Geometry check sheet. Reference: the model listing, model coordinates, mm. A direction names the side the tool comes from. Round coordinates to 2 decimals unless told otherwise and drop trailing zeros. Loops run counter-clockwise (first coordinate to the right, second up) from the corner with the lowest first, then second, coordinate; pieces in that order, holes last.
Autodesk Inventor part; units mm, degrees
ref_plane "YZ Plane" through (0, 0, 0) normal (1, 0, 0) x (0, 1, 0)
ref_plane "XZ Plane" through (0, 0, 0) normal (0, 1, 0) x (-1, 0, 0)
ref_plane "XY Plane" through (0, 0, 0) normal (0, 0, 1) x (1, 0, 0)
sketch "スケッチ1" plane through (0, 0, 0) normal (0, 0, 1) x (1, 0, 0)
  line L0 (0, 0) -> (80, 0)
  line L1 (80, 0) -> (80, 40)
  line L2 (80, 40) -> (0, 40)
  line L3 (0, 40) -> (0, 0)
  dimension "d0" = 80
  dimension "d1" = 40
extrude "押し出し1" add sketch "スケッチ1" along normal blind 40
sketch "スケッチ2" plane through (80, 0, 0) normal (1, 0, 0) x (0, 0, -1)
  line L0 (0, 40) -> (-40, 40)
  line L1 (-37, 40) -> (-3, 40)
  line L2 (-3, 40) -> (-3, 3)
  line L3 (-3, 3) -> (-37, 3)
  line L4 (-37, 3) -> (-37, 40)
  line L5 (-40, 0) -> (-40, 40)
  line L6 (0, 0) -> (0, 40)
  line L7 (0, 0) -> (-40, 0)
  dimension "d4" = 3
  dimension "d5" = 3
  dimension "d6" = 3
extrude "押し出し2" cut sketch "スケッチ2" against normal through all contours L2 L3 L4 L0
sketch "スケッチ3" plane through (0, 0, 40) normal (0, 0, 1) x (1, 0, 0)
  line L0 (0, 40) -> (80, 40)
  line L1 (40, 40) -> (40, 0)
  point P0 (0, 0)
  point P1 (20, 35)
  point P2 (60, 35)
  dimension "d9" = 5
  dimension "d10" = 20
hole "穴1" at (20, 35, 40) at (60, 35, 40) direction (0, 0, -1) diameter 6 end through all
sketch "スケッチ4" plane through (0, 0, 40) normal (0, 0, 1) x (1, 0, 0)
  line L0 (0, 40) -> (80, 40)
  line L1 (40, 40) -> (40, 0)
  point P0 (0, 0)
  point P1 (34, 30)
  point P2 (46, 30)
  dimension "d18" = 6
  dimension "d19" = 10
hole "穴2" at (34, 30, 40) at (46, 30, 40) direction (0, 0, -1) diameter 2.4 end through all
sketch "スケッチ5" plane through (0, 0, 0) normal (0, -1, 0) x (1, 0, 0)
  line L0 (80, 40) -> (0, 40)
  line L1 (40, 40) -> (40, 10)
  point P0 (0, 0)
sketch "スケッチ6" plane through (0, 0, 40) normal (0, 0, 1) x (1, 0, 0)
  line L0 (80, 40) -> (0, 40)
  line L1 (40, 40) -> (40, 0)
  line L2 (0, 0) -> (80, 0)
  circle A0 centre (20, 35) radius 3
  point P0 (20, 5)
  point P1 (60, 5)
  dimension "d27" = 20
  dimension "d28" = 30
hole "穴3" at (20, 5, 40) at (60, 5, 40) direction (0, 0, -1) diameter 2.459 depth 3
sketch "スケッチ7" plane through (0, 0, 0) normal (0, 0, -1) x (-1, 0, 0)
  line L0 (-80, 40) -> (0, 40)
  line L1 (-40, 40) -> (-40, 0)
  line L2 (0, 0) -> (-80, 0)
  circle A0 centre (-60, 35) radius 3
  point P0 (-60, 5)
  point P1 (-20, 5)
  dimension "d36" = 20
  dimension "d37" = 30
hole "穴4" at (60, 5, 0) at (20, 5, 0) direction (0, 0, 1) diameter 2.459 depth 3
sketch "スケッチ8" plane through (0, 0, 0) normal (0, 0, -1) x (-1, 0, 0)
  line L0 (-80, 40) -> (0, 40)
  line L1 (-40, 40) -> (-40, 3)
  line L2 (-80, 3) -> (0, 3)
  point P0 (0, 0)
  point P1 (-72.5, 35)
  point P2 (-7.5, 35)
  dimension "d45" = 5
  dimension "d46" = 32.5
hole "穴5" at (72.5, 35, 0) at (7.5, 35, 0) direction (0, 0, 1) diameter 2.459 depth 3
sketch "スケッチ9" plane through (0, 0, 40) normal (0, 0, 1) x (1, 0, 0)
  circle A0 centre (7.5, 35) radius 1.2295
  circle A1 centre (72.5, 35) radius 1.2295
  point P0 (0, 0)
hole "穴6" at (7.5, 35, 40) at (72.5, 35, 40) direction (0, 0, -1) diameter 2.459 depth 3
properties part number "シリンダーボックス"
1) Sectioned sample at B-B, the plane y = 10. Record the cut outline in (x, z), then the cut area to 3 significant figures.
Report:
outline: (0, 0) - (80, 0) - (80, 3) - (0, 3) - close; (0, 37) - (80, 37) - (80, 40) - (0, 40) - close
area: 480 mm2
2) Scan lines: line 1 along X through (y, z) = (35, 0.75); line 2 along X through (y, z) = (5, 1.9); line 3 along X through (y, z) = (30, 1.4). Record each from-to range of solid material in increasing order.
Report:
line 1: x = 0 to 6.27, 8.73 to 17, 23 to 57, 63 to 71.27, 73.73 to 80
line 2: x = 0 to 18.77, 21.23 to 58.77, 61.23 to 80
line 3: x = 0 to 32.8, 35.2 to 44.8, 47.2 to 80
3) Mould release check, pull along Y, two halves, no side actions. Record for faces 1 (the face through (39, 20, 40)), 2 (the face through (57.97, 37.21, 38.48)): +Y half, -Y half, draft (parallel to the pull), parting line (faces both ways), or undercut.
Report:
face 1: draft
face 2: undercut
4) Sectioned sample at D-D, the plane x = 20. Record the cut outline in (y, z).
Report:
outline: (0, 0) - (3.77, 0) - (3.77, 3) - (3, 3) - (3, 37) - (3.77, 37) - (3.77, 40) - (0, 40) - close; (6.23, 0) - (32, 0) - (32, 3) - (6.23, 3) - close; (6.23, 37) - (32, 37) - (32, 40) - (6.23, 40) - close; (38, 0) - (40, 0) - (40, 3) - (38, 3) - close; (38, 37) - (40, 37) - (40, 40) - (38, 40) - close
5) Sectioned sample at A-A, the plane x = 7.5. Record the cut outline in (y, z).
Report:
outline: (0, 0) - (33.77, 0) - (33.77, 3) - (3, 3) - (3, 37) - (33.77, 37) - (33.77, 40) - (0, 40) - close; (36.23, 0) - (40, 0) - (40, 3) - (36.23, 3) - close; (36.23, 37) - (40, 37) - (40, 40) - (36.23, 40) - close
6) Access from +Z, -Z, +X, -X, +Y, -Y to the whole of each face (thin tool, end or side, straight path). Record for faces 3 (the face through (21.2, 5.27, 38.48)), 4 (the face through (41, 21, 37)).
Report:
face 3: +Z, -Z
face 4: +X, -X, +Y
7) Sectioned sample at C-C, the plane y = 30. Record the cut outline in (x, z).
Report:
outline: (0, 0) - (32.8, 0) - (32.8, 3) - (0, 3) - close; (0, 37) - (32.8, 37) - (32.8, 40) - (0, 40) - close; (35.2, 0) - (44.8, 0) - (44.8, 3) - (35.2, 3) - close; (35.2, 37) - (44.8, 37) - (44.8, 40) - (35.2, 40) - close; (47.2, 0) - (80, 0) - (80, 3) - (47.2, 3) - close; (47.2, 37) - (80, 37) - (80, 40) - (47.2, 40) - close
8) Gauge pin test, flat ends, axial feed: pin 1 (10 mm diameter, centred on x = 14, z = 17, fed in from +Y); pin 2 (3 mm diameter, centred on x = 34, y = 30, fed in from -Z). Record the tip position at first contact, or that the pin passes through.
Report:
pin 1: stops at y = 3
pin 2: stops at z = 0
